For this review, take the finished solid that the model builds, in its own axes (mm). Coordinates: 2 decimals unless noted, no trailing zeros. Loops run counter-clockwise (first coordinate to the right, second up) from the corner with the lowest first, then second, coordinate; pieces in that order, holes last. Notation, with made-up numbers: (72, 63) -> (118, 63) arc R21 cw to (118, 97) -> close; hole circle Ø7 at (-14.75, 16). An arc over 180 degrees is marked (long way). Use a Markdown table: item, result.
from build123d import *

# Parameters (mm, degrees)
SKETCH_1_R      = 3
EXTRUDE_1_DEPTH = 188
SKETCH_2_R      = 2.5
EXTRUDE_2_DEPTH = 41
EXTRUDE_START   = 41
SKETCH_3_R      = 2.5
EXTRUDE_3_DEPTH = 41
CHAMFER_1_SIZE  = 0.5


with BuildPart() as part:
    # 草图1 → 凸台-拉伸1 (new body)
    with BuildSketch(Plane.XY):
        with Locations((-7.816186841, 3.167153776)):
            Circle(SKETCH_1_R)
    extrude(amount=EXTRUDE_1_DEPTH)

    # 草图2 → 凸台-拉伸2 (add)
    with BuildSketch(Plane(origin=(0, 0, 0), x_dir=(-1, 0, 0), z_dir=(0, 0, -1))):
        with Locations(Location((7.816186841, 3.167153776, 0), (0, 0, 180))):
            Circle(SKETCH_2_R)
    extrude(amount=EXTRUDE_2_DEPTH)

    # 草图3 → 凸台-拉伸3 (add)
    with BuildSketch(Plane.XY.offset(188).offset(EXTRUDE_START)):
        with Locations((-7.816186841, 3.167153776)):
            Circle(SKETCH_3_R)
    extrude(amount=-EXTRUDE_3_DEPTH)

    # 倒角1
    chamfer_1_edges = [part.edges().sort_by_distance(p)[0] for p in [
        (-10.316186841, 3.167153776, 229),
        (-10.316186841, 3.167153776, -41),
    ]]
    chamfer(chamfer_1_edges, length=CHAMFER_1_SIZE)


solid = part.part
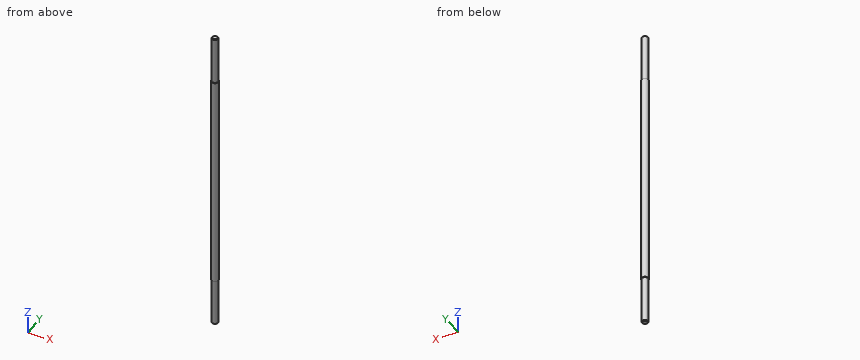
(1) Take a section at A-A on z = 177.5. Write out the cut boundary in (x, y), plus the area to 3 significant figures.
Found:
| item | result |
|---|---|
| outline | circle Ø6 at (-7.82, 3.17) |
| area | 28.3 mm^2 |
(2) For line 1 along X through (y, z) = (0.95, 5.5); line 2 along Z through (x, y) = (-6.1, 5.35); line 3 along X through (y, z) = (3, 163), list the stretches that pass through material, from the lowest coordinate up.
Found:
| item | result |
|---|---|
| line 1 | x = -9.84 to -5.8 |
| line 2 | z = 0 to 188 |
| line 3 | x = -10.81 to -4.82 |
(3) Take a section at B-B on z = -8.5. Write out the cut boundary in (x, y).
Found:
| item | result |
|---|---|
| outline | circle Ø5 at (-7.82, 3.17) |
(4) For pin 1 Ø1 at (x, y) = (-6, 5) entering from +Z; pin 2 Ø2 at (x, z) = (-10, 180) entering from -Y, all flat-tipped, find the tip position at first contact; note any pin that passes through.
Found:
| item | result |
|---|---|
| pin 1 | stops at z = 228.92 |
| pin 2 | stops at y = 0.41 |
